The model under review builds one solid part; all positions refer to its coordinate system, in mm. A direction names the side the tool comes from. Round coordinates to 2 decimals unless told otherwise and drop trailing zeros. Write each loop counter-clockwise with the first axis right and the second up, starting at its lowest first coordinate (ties: lowest second). Pieces come first, ordered by that corner, then holes.
Item 1: Add section D-D (y = -26). Give the boundary of the cut face in (x, z).
Item 2: Add section C-C (z = 3.5). Give the boundary of the cut face in (x, y).
Item 3: Add section A-A (y = 0). Give the boundary of the cut face in (x, z).
Item 4: Clearance check with flat-ended pins moving along their axes: pin 1 Ø11.5 at (y, z) = (0, 0) entering from -X; pin 2 Ø8 at (x, y) = (2.5, -6) entering from -Z; pin 3 Ø12 at (y, z) = (-7.5, 11.5) entering from +X; pin 4 Ø8 at (x, z) = (9, -13) entering from +Y. State where each tip first meets the part, or that it passes through.
Item 5: Add section B-B (x = 36.5). Give the boundary of the cut face in (y, z), plus the area to 3 significant figures.
Item 6: To check wall thickness, follow L1, parallel to X at y = -20, z = 27; L2, parallel to X at y = -13, z = -3; L3, parallel to Z at x = 33, y = -10.5. State the ranges of each line that lie inside material, in increasing order.
Item 7: Draft analysis for pull direction Y (two halves, no side actions). For faces 6 (the face through (0, -5, 11)), 7 (the face through (14, -30, 11)), 8 (the face through (5, 20, 20)), 9 (the face through (4.93, -4.88, 1.08)), state which applies: +Y half, -Y half, draft (parallel to the pull), parting line (faces both ways), or undercut.
Item 8: Machinability: for faces 1 (the face through (20, -22, 5)), 2 (the face through (25, -10, 25)), 3 (the face through (10, -20, -15)), 4 (the face through (19.1, -10.2, 30)), 5 (the face through (15, -15, 5)), which of the approach directions +Z, -Z, +X, -X, +Y, -Y give a long, thin tool a straight path to every point of the face, cutting with its end or side? Answer none if there is none.
```python
from build123d import *

# Parameters (mm, degrees)
SKETCH1_W           = 10
SKETCH1_H           = 20
BOSS_EXTRUDE1_DEPTH = 50
SKETCH1_3_W         = 10
SKETCH1_3_H         = 10
BOSS_EXTRUDE2_DEPTH = 20
SKETCH1_4_R         = 5
BOSS_EXTRUDE3_DEPTH = 10
FILLET1_R           = 10
SKETCH2_R           = 5
CUT_EXTRUDE1_DEPTH  = 10


with BuildPart() as part:
    # Sketch1 → Boss-Extrude1 (new body)
    with BuildSketch(Plane(origin=(0, 0, 0), x_dir=(0, 0, -1), z_dir=(1, 0, 0))):
        with Locations((-25, -20)):
            Rectangle(SKETCH1_W, SKETCH1_H)
    extrude(amount=BOSS_EXTRUDE1_DEPTH)

    # Sketch1_3 → Boss-Extrude2 (add)
    with BuildSketch(Plane(origin=(0, 0, 0), x_dir=(0, 0, -1), z_dir=(1, 0, 0))):
        Polygon((10, -20), (-20, -10), (-20, -30), (10, -30), align=None)
        with Locations((15, -25)):
            Rectangle(SKETCH1_3_W, SKETCH1_3_H)
    extrude(amount=BOSS_EXTRUDE2_DEPTH)

    # Sketch1_4 → Boss-Extrude3 (add)
    with BuildSketch(Plane(origin=(0, 0, 0), x_dir=(0, 0, -1), z_dir=(1, 0, 0))):
        Polygon((-10, 20), (-30, 20), (-30, -10), (-20, -10), (10, -20), (10, 10), align=None)
        Circle(SKETCH1_4_R, mode=Mode.SUBTRACT)
    extrude(amount=BOSS_EXTRUDE3_DEPTH)

    # Fillet1
    fillet1_edges = [part.edges().sort_by_distance(p)[0] for p in [
        (50, -10, 25),
        (20, -25, -20),
    ]]
    fillet(fillet1_edges, radius=FILLET1_R)

    # Sketch2 → Cut-Extrude1 (cut)
    with BuildSketch(Plane(origin=(0, 0, 20), x_dir=(-1, 0, 0), z_dir=(0, 0, -1))):
        with Locations(Location((-40, -20, 0), (0, 0, 90))):
            Circle(SKETCH2_R)
    extrude(amount=-CUT_EXTRUDE1_DEPTH, mode=Mode.SUBTRACT)


solid = part.part
```
Numbers:
1. outline: (0, -20) - (10, -20) arc R10 ccw to (20, -10) - (20, 20) - (50, 20) - (50, 30) - (0, 30) - close
2. outline: (0, -30) - (20, -30) - (20, -15.5) - (10, -15.5) - (10, -3.57) - (0, -3.57) - close; (0, 3.57) - (10, 3.57) - (10, 16.75) - (0, 16.75) - close
3. outline: (0, -10) - (10, -10) - (10, -5) - (0, -5) - close; (0, 5) - (10, 5) - (10, 30) - (0, 30) - close
4. pin 1: stops at x = 0
4. pin 2: stops at z = -10
4. pin 3: stops at x = 20
4. pin 4: stops at y = 10.5
5. outline: (-30, 20) - (-23.57, 20) - (-23.57, 30) - (-30, 30) - close; (-16.43, 20) - (-10, 20) - (-10, 30) - (-16.43, 30) - close
5. area: 129 mm2
6. L1: x = 0 to 35, 45 to 50
6. L2: x = 0 to 10
6. L3: z = 20 to 30
7. face 6: draft
7. face 7: -Y half
7. face 8: +Y half
7. face 9: undercut
8. face 1: -Z, +X, +Y, -Y
8. face 2: +Z, -Z, +X, +Y
8. face 3: -Z, +X, -X, +Y
8. face 4: +Z, +X, -X, +Y, -Y
8. face 5: -Z, +X, +Y
